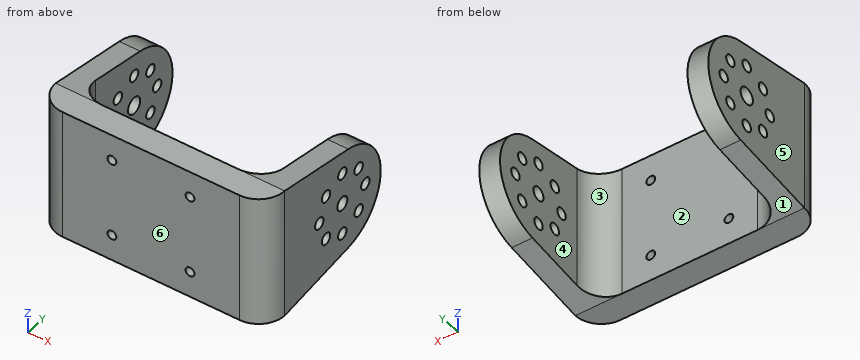
from build123d import *

# Parameters (mm, degrees)
SKETCH_1_W          = 44
SKETCH_1_H          = 25
EXTRUDE_1_DEPTH     = 5
SKETCH_2_R          = 1.1
SKETCH_2_R_2        = 1.6
EXTRUDE_2_DEPTH     = 4
EXTRUDE_START       = -4
SKETCH_3_R          = 1.3
SKETCH_3_R_2        = 1.1
EXTRUDE_3_DEPTH     = 4
FILLET_1_R          = 5
SKETCH_4_R          = 0.85
CUT_EXTRUDE_1_DEPTH = 5


with BuildPart() as part:
    # ｽｹｯﾁ1 → ﾎﾞｽ - 押し出し1 (new body)
    with BuildSketch(Plane(origin=(0, 0, 0), x_dir=(1, 0, 0), z_dir=(0, 1, 0))):
        with Locations((0, 12.5)):
            Rectangle(SKETCH_1_W, SKETCH_1_H)
    extrude(amount=EXTRUDE_1_DEPTH)

    # ｽｹｯﾁ2 → ﾎﾞｽ - 押し出し2 (add)
    with BuildSketch(Plane.ZY.offset(22)):
        with BuildLine():
            Line((-25, 5), (0, 5))
            Line((0, 5), (-2.623078099, 21.564101584))
            ThreePointArc((-2.623078099, 21.564101584), (-12.5, 30), (-22.376921901, 21.564101584))
            Line((-22.376921901, 21.564101584), (-25, 5))
        make_face()
        with Locations((-12.5, 26)):
            Circle(SKETCH_2_R, mode=Mode.SUBTRACT)
        with Locations((-8.257359313, 24.242640687)):
            Circle(SKETCH_2_R, mode=Mode.SUBTRACT)
        with Locations((-6.5, 20)):
            Circle(SKETCH_2_R, mode=Mode.SUBTRACT)
        with Locations((-8.257359313, 15.757359313)):
            Circle(SKETCH_2_R, mode=Mode.SUBTRACT)
        with Locations((-12.5, 14)):
            Circle(SKETCH_2_R, mode=Mode.SUBTRACT)
        with Locations((-16.742640687, 15.757359313)):
            Circle(SKETCH_2_R, mode=Mode.SUBTRACT)
        with Locations((-18.5, 20)):
            Circle(SKETCH_2_R, mode=Mode.SUBTRACT)
        with Locations((-16.742640687, 24.242640687)):
            Circle(SKETCH_2_R, mode=Mode.SUBTRACT)
        with Locations((-12.5, 20)):
            Circle(SKETCH_2_R_2, mode=Mode.SUBTRACT)
    extrude(amount=-EXTRUDE_2_DEPTH)

    # ｽｹｯﾁ3 → ﾎﾞｽ - 押し出し3 (add)
    with BuildSketch(Plane(origin=(22, 0, 0), x_dir=(0, 0, -1), z_dir=(1, 0, 0)).offset(EXTRUDE_START)):
        with BuildLine():
            Line((0, 5), (2.623078099, 21.564101584))
            ThreePointArc((2.623078099, 21.564101584), (12.5, 30), (22.376921901, 21.564101584))
            Line((22.376921901, 21.564101584), (25, 5))
            Line((25, 5), (0, 5))
        make_face()
        with Locations((12.5, 20)):
            Circle(SKETCH_3_R, mode=Mode.SUBTRACT)
        with Locations(Location((8.257359313, 15.757359313, 0), (0, 0, 180))):
            Circle(SKETCH_3_R_2, mode=Mode.SUBTRACT)
        with Locations(Location((12.5, 14, 0), (0, 0, 180))):
            Circle(SKETCH_3_R_2, mode=Mode.SUBTRACT)
        with Locations(Location((16.742640687, 15.757359313, 0), (0, 0, 180))):
            Circle(SKETCH_3_R_2, mode=Mode.SUBTRACT)
        with Locations(Location((18.5, 20, 0), (0, 0, 180))):
            Circle(SKETCH_3_R_2, mode=Mode.SUBTRACT)
        with Locations(Location((16.742640687, 24.242640687, 0), (0, 0, 180))):
            Circle(SKETCH_3_R_2, mode=Mode.SUBTRACT)
        with Locations(Location((12.5, 26, 0), (0, 0, 180))):
            Circle(SKETCH_3_R_2, mode=Mode.SUBTRACT)
        with Locations(Location((8.257359313, 24.242640687, 0), (0, 0, 180))):
            Circle(SKETCH_3_R_2, mode=Mode.SUBTRACT)
        with Locations(Location((6.5, 20, 0), (0, 0, 180))):
            Circle(SKETCH_3_R_2, mode=Mode.SUBTRACT)
    extrude(amount=EXTRUDE_3_DEPTH)

    # ﾌｨﾚｯﾄ1
    fillet_1_edges = [part.edges().sort_by_distance(p)[0] for p in [
        (18, 5, -12.5),
        (-18, 5, -12.5),
        (22, 0, -12.5),
        (-22, 0, -12.5),
    ]]
    fillet(fillet_1_edges, radius=FILLET_1_R)

    # ｽｹｯﾁ4 → ｶｯﾄ - 押し出し1 (cut)
    with BuildSketch(Plane(origin=(0, 5, 0), x_dir=(1, 0, 0), z_dir=(0, 1, 0))):
        with Locations(Location((-7.5, 20, 0), (0, 0, 270))):
            Circle(SKETCH_4_R)
        with Locations(Location((7.5, 20, 0), (0, 0, 270))):
            Circle(SKETCH_4_R)
        with Locations(Location((7.5, 5, 0), (0, 0, 270))):
            Circle(SKETCH_4_R)
        with Locations(Location((-7.5, 5, 0), (0, 0, 270))):
            Circle(SKETCH_4_R)
    extrude(amount=-CUT_EXTRUDE_1_DEPTH, mode=Mode.SUBTRACT)


solid = part.part
Here's how the part is built. I have some questions about the finished solid (model axes, mm). Face numbers are marked on the shaded views. A direction names the side the tool comes from. Round coordinates to 2 decimals unless told otherwise and drop trailing zeros. Order: outer loops, then holes, each group sorted by start corner. A loop starts at its lowest first (then second) coordinate and runs counter-clockwise, first axis right, second up. Notation, with made-up numbers: M -11,34.25 L 35,34.25 A17 cw 35,39.25 Z; hole C 36,-19.5 d11. An arc over 180 degrees is marked long. Return JSON: item names as keys, results as strings. Group by question number.
1. If we section it at D-D on y = 20: State how many separate pieces and enclosed holes the cut face has, then the cut area to 3 significant figures.
2. If we section it at C-C on z = -16.75: List the corners of the cut face in (x, y) for me.
3. Please list where these lines run through material, in increasing order: probe 1 along X at (y, z) = (13, -5.75); probe 2 along Y at (x, z) = (19.55, -12.5); probe 3 along Y at (x, z) = (20.9, -12.5).
4. If we mould it in two halves opening along X, with no side actions, what happens to the marked faces 3, 4, 5 and 6? For each: pulls with the +X half, pulls with the -X half, needs draft (parallel to the pull), parting line crosses it, or undercut.
5. On a 3-axis mill with a long thin cutter (end or side, diameter ignored), from which of +Z, -Z, +X, -X, +Y, -Y can I reach the whole of each face in a straight line? I mean the marked faces 1 and 2. Say none if no direction works.
6. If we section it at A-A on z = -6.5: List the corners of the cut face in (x, y) for me, then the cut area to 3 significant figures.
7. If we section it at B-B on y = 6.75: List the corners of the cut face in (x, z) for me.
8. I'm going to push flat-ended pins straight in: pin 1 Ø1.5 at (x, z) = (-5.5, -11) entering from +Y; pin 2 Ø2 at (x, z) = (15, -19) entering from +Y. Where does each tip first touch, or does it pass through?
Reply:
{
 "1": {"separate pieces": "8", "enclosed holes": "0", "area": "104 mm^2"},
 "2": {"outline": "M -22,5 A5 ccw -17,0 L 17,0 A5 ccw 22,5 L 22,14.66 L 18,14.66 L 18,10 A5 cw 13,5 L -13,5 A5 cw -18,10 L -18,14.66 L -22,14.66 Z; M -22,16.86 L -18,16.86 L -18,23.14 L -22,23.14 Z; M -22,25.34 L -18,25.34 L -18,29.05 L -22,29.05 Z; M 18,16.86 L 22,16.86 L 22,23.14 L 18,23.14 Z; M 18,25.34 L 22,25.34 L 22,29.05 L 18,29.05 Z"},
 "3": {"probe 1": "-22 to -18, 18 to 22", "probe 2": "0.7 to 12.9, 15.1 to 18.7, 21.3 to 24.9, 27.1 to 30", "probe 3": "1.87 to 12.9, 15.1 to 18.7, 21.3 to 24.9, 27.1 to 30"},
 "4": {"face 3": "undercut", "face 4": "undercut", "face 5": "pulls with the -X half", "face 6": "needs draft"},
 "5": {"face 1": "-Z, +X, -X, +Y", "face 2": "+Z, -Z, +Y"},
 "6": {"outline": "M -22,5 A5 ccw -17,0 L 17,0 A5 ccw 22,5 L 22,18.9 L 18,18.9 L 18,10 A5 cw 13,5 L -13,5 A5 cw -18,10 L -18,18.9 L -22,18.9 Z; M -22,21.1 L -18,21.1 L -18,28 L -22,28 Z; M 18,21.1 L 22,21.1 L 22,28 L 18,28 Z", "area": "386 mm^2"},
 "7": {"outline": "M -22,-24.72 L -16.8,-24.72 L -16.8,-0.28 L -22,-0.28 Z; M 16.8,-24.72 L 22,-24.72 L 22,-0.28 L 16.8,-0.28 Z"},
 "8": {"pin 1": "y = 5", "pin 2": "y = 6"}
}
